Check sheet for the modelled part. Datum: model origin and axes. Units: mm. A direction names the side the tool comes from. Give positions to 0.01 mm unless a question says otherwise; leave off trailing zeros. Order: outer loops, then holes, each group sorted by start corner. A loop starts at its lowest first (then second) coordinate and runs counter-clockwise, first axis right, second up.
from build123d import *

# Parameters (mm, degrees)
F0_W      = 19.8374
F0_H      = 24.9936
F1_DEPTH  = 14.8336
F2_R      = 2.9591
F2_R_2    = 0.9906
F3_DEPTH  = 1.6764
F3_FACE_R = 0.9906
F4_DEPTH  = 8.9662
F5_R      = 6.132102
F6_R      = 0.9779
F7_DEPTH  = 2.032
F7_FACE_R = 0.9779
F8_DEPTH  = 3.302
F9_R      = 2.667
F10_DEPTH = 5.334


with BuildPart() as f1:
    # F0 (on Top) → F1 (new body)
    with BuildSketch(Plane.XY):
        with Locations((-0.465175, 7.303395)):
            Rectangle(F0_W, F0_H)
    extrude(amount=F1_DEPTH)

    # F2 (on face) → F3 (join)
    with BuildSketch(Plane.XZ.offset(5.193405)):
        with Locations((0, 7.4168)):
            Circle(F2_R)
        with Locations((0, 7.4168)):
            Circle(F2_R_2, mode=Mode.SUBTRACT)
    extrude(amount=F3_DEPTH)

    # F3_face (on face) → F4 (join)
    with BuildSketch(Plane(origin=(0, -5.193405, 7.4168), x_dir=(1, 0, 0), z_dir=(0, -1, 0))):
        Circle(F3_FACE_R)
    extrude(amount=F4_DEPTH)

    # F5
    f5_edges = [f1.edges().sort_by_distance(p)[0] for p in [
        (9.453525, 7.303395, 14.8336),
        (9.453525, 7.303395, 0),
        (-10.383875, 7.303395, 14.8336),
        (-10.383875, 7.303395, 0),
    ]]
    fillet(f5_edges, radius=F5_R)

    # F6 (on face) → F7 (join)
    with BuildSketch(Plane(origin=(0, 19.800195, 0), x_dir=(-1, 0, 0), z_dir=(0, 1, 0))):
        with BuildLine():
            ThreePointArc((-3.009659, 11.3665), (-2.20376, 2.966899), (4.9657, 7.4168))
            ThreePointArc((4.9657, 7.4168), (4.449901, 9.62056), (3.009659, 11.3665))
            Line((3.009659, 11.3665), (-3.009659, 11.3665))
        make_face()
        with Locations((0, 7.4168)):
            Circle(F6_R, mode=Mode.SUBTRACT)
    extrude(amount=F7_DEPTH)

    # F7_face (on face) → F8 (join)
    with BuildSketch(Plane(origin=(0, 19.800195, 7.4168), x_dir=(-1, 0, 0), z_dir=(0, 1, 0))):
        Circle(F7_FACE_R)
    extrude(amount=F8_DEPTH)

    # F9 (on face) → F10 (cut)
    with BuildSketch(Plane(origin=(0, 19.800195, 0), x_dir=(-1, 0, 0), z_dir=(0, 1, 0))):
        with Locations((-9.453525, 7.4168)):
            Circle(F9_R)
        with Locations((10.383875, 7.4168)):
            Circle(F9_R)
    extrude(amount=-F10_DEPTH, mode=Mode.SUBTRACT)


solid = f1.part
1) Section check C-C, the plane z = 3.75. Record the cut outline in (x, y), then the cut area to 3 significant figures.
Recorded:
outline: (-9.9, -5.19) - (8.97, -5.19) - (8.97, 19.8) - (3.35, 19.8) - (3.35, 21.83) - (-3.35, 21.83) - (-3.35, 19.8) - (-9.9, 19.8) - close
area: 485 mm2
2) Depth check by flat-ended pin: pin 1 Ø0.6 at (x, y) = (1, 20.5) entering from +Z; pin 2 Ø3 at (x, z) = (-5, 3.5) entering from +Y; pin 3 Ø3 at (x, z) = (-8.5, 8) entering from +Y. Enter the tip coordinate at first touch or a pass-through.
Recorded:
pin 1: stops at z = 11.37
pin 2: stops at y = 21.83
pin 3: stops at y = 19.8
3) Section check A-A, the plane y = 19. Record the cut outline in (x, z), then the cut area to 3 significant figures.
Recorded:
outline: (-10.23, 4.75) arc R6.13 ccw to (-4.25, 0) - (3.32, 0) arc R6.13 ccw to (9.3, 4.75) arc R2.67 cw to (9.3, 10.08) arc R6.13 ccw to (3.32, 14.83) - (-4.25, 14.83) arc R6.13 ccw to (-10.23, 10.08) arc R2.67 cw to start
area: 240 mm2
4) Set-up check for faces 4 (the face through (6.787, 17.171, 7.36)), 5 (the face through (0.21, 22.46, 6.46)), 6 (the face through (0, -14.16, 7)), 7 (the face through (1.3, -6.87, 7.5)), 8 (the face through (0, 21, 11.366)): record each of +Z, -Z, +X, -X, +Y, -Y from which the full face is reachable in a straight line by a thin tool's end or side.
Recorded:
face 4: +X, +Y
face 5: +Y
face 6: +Z, -Z, +X, -X, -Y
face 7: -Y
face 8: +Z, +X, -X, +Y
5) Section check D-D, the plane z = 12.75. Record the cut outline in (x, y), then the cut area to 3 significant figures.
Recorded:
outline: (-8.86, -5.19) - (7.93, -5.19) - (7.93, 19.8) - (-8.86, 19.8) - close
area: 420 mm2
6) Material ranges on L1, parallel to Y at x = 2, z = 2.5; L2, parallel to Y at x = -3, z = 7; L3, parallel to X at y = -10, z = 7.5, recorded low to high.
Recorded:
L1: y = -5.19 to 19.8
L2: y = -5.19 to 21.83
L3: x = -0.99 to 0.99
7) Draft check along Z on faces 1 (the face through (-7.717, 17.171, 7.473)), 2 (the face through (-5, 19.8, 6)), 3 (the face through (7.61, 7.48, 1.75)). Enter one of: +Z half, -Z half, draft (parallel to the pull), parting line (faces both ways), or undercut.
Recorded:
face 1: undercut
face 2: draft
face 3: -Z half
8) Section check B-B, the plane x = 0. Record the cut outline in (y, z).
Recorded:
outline: (-14.16, 6.43) - (-6.87, 6.43) - (-6.87, 4.46) - (-5.19, 4.46) - (-5.19, 0) - (19.8, 0) - (19.8, 2.45) - (21.83, 2.45) - (21.83, 6.44) - (23.1, 6.44) - (23.1, 8.39) - (21.83, 8.39) - (21.83, 11.37) - (19.8, 11.37) - (19.8, 14.83) - (-5.19, 14.83) - (-5.19, 10.38) - (-6.87, 10.38) - (-6.87, 8.41) - (-14.16, 8.41) - close
